Check sheet for the drawn part. Datum: minimum x, y, z corner. Units: mm. Coordinates: 2 decimals unless noted, no trailing zeros. Order: outer loops, then holes, each group sorted by start corner. A loop starts at its lowest first (then second) coordinate and runs counter-clockwise, first axis right, second up. Notation, with made-up numbers: M -26.5,71.5 L -22.5,71.5 A33 ccw -22.5,105.5 Z; hole C 38,37 d8. An arc over 180 degrees is marked long. Return JSON: item names as keys, results as strings. Group by question number.
Q1. Section check B-B, the plane x = 127.5. Enter the section's corners in (y, z).
Q2. Go/stop test with a flat-tipped pin: pin 1 Ø4 at (x, y) = (138, 12) entering from +Z. Record where the tip stops, or that it passes through.
Q3. Section check A-A, the plane y = 12. Enter the section's corners in (x, z), then the cut area to 3 significant figures.
Q4. Thickness scan on probe 1 along Y at (x, z) = (138, 4); probe 2 along X at (y, z) = (87.5, 2). Record the ranges inside material, lowest first.
Q5. Section check C-C, the plane z = 2.25. Enter the section's corners in (x, y).
Q6. Section check D-D, the plane y = 59. Enter the section's corners in (x, z), then the cut area to 3 significant figures.
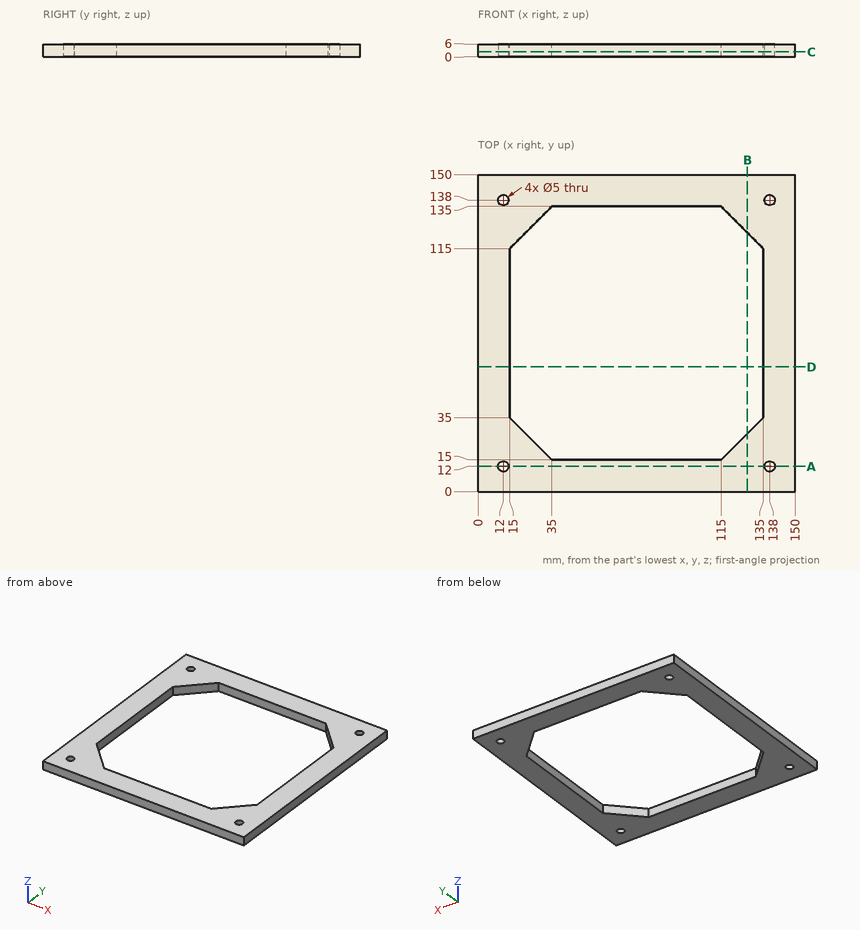
Numbers:
{
 "1": {"outline": "M 0,0 L 27.5,0 L 27.5,6 L 0,6 Z; M 122.5,0 L 150,0 L 150,6 L 122.5,6 Z"},
 "2": {"pin 1": "passes through"},
 "3": {"outline": "M 0,0 L 9.5,0 L 9.5,6 L 0,6 Z; M 14.5,0 L 135.5,0 L 135.5,6 L 14.5,6 Z; M 140.5,0 L 150,0 L 150,6 L 140.5,6 Z", "area": "840 mm2"},
 "4": {"probe 1": "y = 0 to 9.5, 14.5 to 135.5, 140.5 to 150", "probe 2": "x = 0 to 15, 135 to 150"},
 "5": {"outline": "M 0,0 L 150,0 L 150,150 L 0,150 Z; hole C 12,12 d5; hole C 12,138 d5; hole M 15,35 L 35,15 L 115,15 L 135,35 L 135,115 L 115,135 L 35,135 L 15,115 Z; hole C 138,12 d5; hole C 138,138 d5"},
 "6": {"outline": "M 0,0 L 15,0 L 15,6 L 0,6 Z; M 135,0 L 150,0 L 150,6 L 135,6 Z", "area": "180 mm2"}
}
